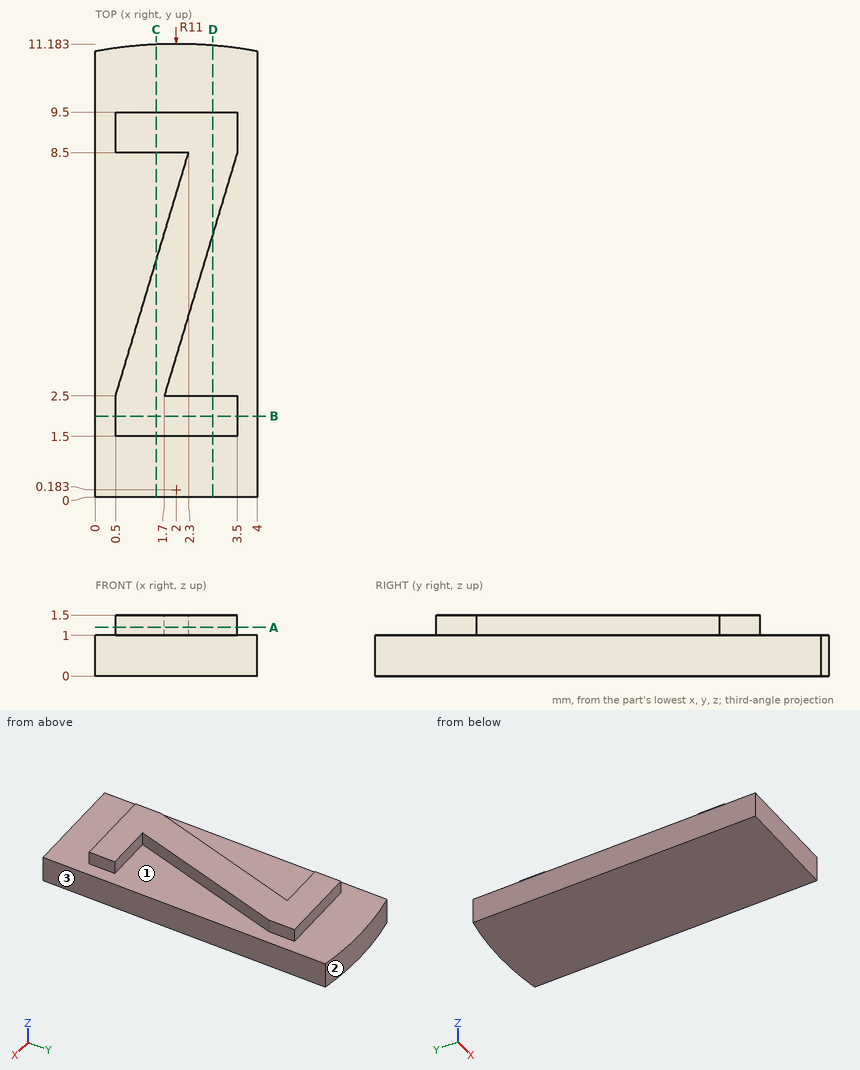
Input: dimensioned drawing with shaded views. Units: mm. Origin: part minimum x, y, z. Coordinates: 2 decimals unless noted, no trailing zeros. Order: outer loops, then holes, each group sorted by start corner. A loop starts at its lowest first (then second) coordinate and runs counter-clockwise, first axis right, second up.
1. Cut plane A-A, the plane z = 1.2. Return loops of the section in (x, y).
Checked values:
outline: (0.5, 1.5) - (3.5, 1.5) - (3.5, 2.5) - (1.7, 2.5) - (3.5, 8.5) - (3.5, 9.5) - (0.5, 9.5) - (0.5, 8.5) - (2.3, 8.5) - (0.5, 2.5) - close
2. Cut plane D-D, the plane x = 2.9. Return loops of the section in (y, z).
Checked values:
outline: (0, 0) - (11.15, 0) - (11.15, 1) - (9.5, 1) - (9.5, 1.5) - (6.5, 1.5) - (6.5, 1) - (2.5, 1) - (2.5, 1.5) - (1.5, 1.5) - (1.5, 1) - (0, 1) - close
3. Contact query for a flat-ended pin moving along its axis: P1, Ø0.6, axis at x = 3, z = 1.5, coming from the +Y side. Output: stop coordinate, or through.
Checked values:
P1: stops at y = 9.5
4. Cut plane B-B, the plane y = 2. Return loops of the section in (x, z).
Checked values:
outline: (0, 0) - (4, 0) - (4, 1) - (3.5, 1) - (3.5, 1.5) - (0.5, 1.5) - (0.5, 1) - (0, 1) - close
5. Draft query along Y for the marked faces 1, 2 and 3. Return one class per face: +Y half, -Y half, draft (parallel to the pull), parting line (faces both ways), or undercut.
Checked values:
face 1: undercut
face 2: +Y half
face 3: draft
6. Ray query, line 1 along Z through (x, y) = (3.65, 8); line 2 along X through (y, z) = (9, 1.25); line 3 along X through (y, z) = (5.25, 1.3) (1 decimal). Return the intervals inside material, ascending.
Checked values:
line 1: z = 0 to 1
line 2: x = 0.5 to 3.5
line 3: x = 1.3 to 2.5
7. Cut plane C-C, the plane x = 1.5. Return loops of the section in (y, z).
Checked values:
outline: (0, 0) - (11.17, 0) - (11.17, 1) - (9.5, 1) - (9.5, 1.5) - (8.5, 1.5) - (8.5, 1) - (5.83, 1) - (5.83, 1.5) - (1.5, 1.5) - (1.5, 1) - (0, 1) - close
